Can you work these out from the model? Positions are in its coordinate system, mm. Face numbers are marked on the shaded views. A direction names the side the tool comes from. Round coordinates to 2 decimals unless told otherwise and drop trailing zeros. Loops run counter-clockwise (first coordinate to the right, second up) from the corner with the lowest first, then second, coordinate; pieces in that order, holes last. Notation, with made-up numbers: (-2, 53.25) -> (55, 53.25) arc R15 ccw to (55, 66.25) -> close; hole circle Ø2 at (-18.5, -34.5). An arc over 180 degrees is marked (long way). Answer as a JSON object with one key per item and string values.
```python
from build123d import *

# Parameters (mm, degrees)
EXTRUDE_1_DEPTH   = 10
EXTRUDE_1_2_DEPTH = 10
EXTRUDE_1_3_DEPTH = 10
SKETCH_1_3_R      = 25
SKETCH_1_3_R_2    = 7.5
SKETCH_1_3_R_3    = 5
SKETCH_1_3_R_4    = 43
SKETCH_1_3_R_5    = 6
SKETCH_1_3_R_6    = 16
EXTRUDE_2_DEPTH   = 20


with BuildPart() as part:
    # Sketch 1 → Extrude 1 (new body)
    with BuildSketch(Plane.XY):
        with BuildLine():
            ThreePointArc((105.256123955, 41.758974142), (43.471517996, 43.816308869), (-13.895789474, 20.782373178))
            ThreePointArc((-13.895789474, 20.782373178), (3.574397154, 24.743154306), (19.209372712, 16))
            ThreePointArc((19.209372712, 16), (18.448719356, 19.393999935), (20.761928319, 21.991478208))
            ThreePointArc((20.761928319, 21.991478208), (36.009186006, 26.873359096), (51.727153653, 29.915910824))
            ThreePointArc((51.727153653, 29.915910824), (57.357710528, 27.382727589), (57.596791581, 21.213203436))
            ThreePointArc((57.596791581, 21.213203436), (77.977273362, 39.487045696), (105.256123955, 41.758974142))
        make_face()
    extrude(amount=EXTRUDE_1_DEPTH)



with BuildPart() as body_2:
    # Sketch 1 → Extrude 1 2 (new body)
    with BuildSketch(Plane.XY):
        with BuildLine():
            ThreePointArc((47.755952756, -7), (51.392501916, -8.227630546), (53.540938133, -11.408163265))
            ThreePointArc((53.540938133, -11.408163265), (52, 0), (53.540938133, 11.408163265))
            ThreePointArc((53.540938133, 11.408163265), (51.392501916, 8.227630546), (47.755952756, 7))
            Line((47.755952756, 7), (28.142494559, 7))
            ThreePointArc((28.142494559, 7), (24.909599122, 7.945458765), (22.695560128, 10.483870968))
            ThreePointArc((22.695560128, 10.483870968), (24.417094455, 5.367075405), (25, 0))
            ThreePointArc((25, 0), (24.417094455, -5.367075405), (22.695560128, -10.483870968))
            ThreePointArc((22.695560128, -10.483870968), (24.909599122, -7.945458765), (28.142494559, -7))
            Line((28.142494559, -7), (47.755952756, -7))
        make_face()
    extrude(amount=EXTRUDE_1_2_DEPTH)


with BuildPart() as body_3:
    # Sketch 1 → Extrude 1 3 (new body)
    with BuildSketch(Plane.XY):
        with BuildLine():
            ThreePointArc((-54, 29), (-58.686291501, 40.313708499), (-70, 45))
            Line((-70, 45), (-70, -125))
            ThreePointArc((-70, -125), (-58.686291501, -120.313708499), (-54, -109))
            Line((-54, -109), (-54, -100.391329163))
            ThreePointArc((-54, -100.391329163), (-51.241745904, -92.047280445), (-44.053835854, -86.991089805))
            Line((-44.053835854, -86.991089805), (107.451067266, -41.15787803))
            ThreePointArc((107.451067266, -41.15787803), (81.540043629, -40.839069217), (60.517137347, -25.689145242))
            ThreePointArc((60.517137347, -25.689145242), (61.99532492, -34.793587478), (55.393464002, -41.234964608))
            Line((55.393464002, -41.234964608), (14.737358223, -53.534235903))
            ThreePointArc((14.737358223, -53.534235903), (9.423979121, -52.60916728), (7, -47.791276178))
            Line((7, -47.791276178), (7, -28.142494559))
            ThreePointArc((7, -28.142494559), (7.945458765, -24.909599122), (10.483870968, -22.695560128))
            ThreePointArc((10.483870968, -22.695560128), (0, -25), (-10.483870968, -22.695560128))
            ThreePointArc((-10.483870968, -22.695560128), (-7.945458765, -24.909599122), (-7, -28.142494559))
            Line((-7, -28.142494559), (-7, -55.656787337))
            ThreePointArc((-7, -55.656787337), (-8.182108898, -59.232808217), (-11.262641777, -61.399747063))
            Line((-11.262641777, -61.399747063), (-41.104402961, -70.427466509))
            ThreePointArc((-41.104402961, -70.427466509), (-49.960034799, -68.88568547), (-54, -60.855866967))
            Line((-54, -60.855866967), (-54, -13.5))
            ThreePointArc((-54, -13.5), (-52.242640687, -9.257359313), (-48, -7.5))
            Line((-48, -7.5), (-27.906092525, -7.5))
            ThreePointArc((-27.906092525, -7.5), (-24.718414636, -8.416820908), (-22.504913326, -10.887096774))
            ThreePointArc((-22.504913326, -10.887096774), (-25, 0), (-22.504913326, 10.887096774))
            ThreePointArc((-22.504913326, 10.887096774), (-24.718414636, 8.416820908), (-27.906092525, 7.5))
            Line((-27.906092525, 7.5), (-48, 7.5))
            ThreePointArc((-48, 7.5), (-52.242640687, 9.257359313), (-54, 13.5))
            Line((-54, 13.5), (-54, 29))
        make_face()
    extrude(amount=EXTRUDE_1_3_DEPTH)


with BuildPart() as part_1:
    add(part.part)

    add(body_2.part)  # Extrude 2 merges body 2

    add(body_3.part)  # Extrude 2 merges body 3
    # Sketch 1_3 → Extrude 2 (add)
    # profile 1 of 2: a face of its own
    with BuildSketch(Plane.XY):
        with Locations(Location((0, 0, 0), (0, 0, 154.183912666))):
            Circle(SKETCH_1_3_R)
        Circle(SKETCH_1_3_R_2, mode=Mode.SUBTRACT)
        with Locations((0, 16)):
            Circle(SKETCH_1_3_R_3, mode=Mode.SUBTRACT)
        with Locations((13.856406461, -8)):
            Circle(SKETCH_1_3_R_3, mode=Mode.SUBTRACT)
        with Locations((-13.856406461, -8)):
            Circle(SKETCH_1_3_R_3, mode=Mode.SUBTRACT)
    # profile 2 of 2: a face of its own
    with BuildSketch(Plane.XY):
        with Locations(Location((95, 0, 0), (0, 0, 164.614856568))):
            Circle(SKETCH_1_3_R_4)
        with Locations((73.786796564, 21.213203436)):
            Circle(SKETCH_1_3_R_5, mode=Mode.SUBTRACT)
        with Locations((65, 0)):
            Circle(SKETCH_1_3_R_5, mode=Mode.SUBTRACT)
        with Locations((73.786796564, -21.213203436)):
            Circle(SKETCH_1_3_R_5, mode=Mode.SUBTRACT)
        with Locations((95, -30)):
            Circle(SKETCH_1_3_R_5, mode=Mode.SUBTRACT)
        with Locations((116.213203436, -21.213203436)):
            Circle(SKETCH_1_3_R_5, mode=Mode.SUBTRACT)
        with Locations((125, 0)):
            Circle(SKETCH_1_3_R_5, mode=Mode.SUBTRACT)
        with Locations((116.213203436, 21.213203436)):
            Circle(SKETCH_1_3_R_5, mode=Mode.SUBTRACT)
        with Locations((95, 30)):
            Circle(SKETCH_1_3_R_5, mode=Mode.SUBTRACT)
        with Locations((95, 0)):
            Circle(SKETCH_1_3_R_6, mode=Mode.SUBTRACT)
    extrude(amount=EXTRUDE_2_DEPTH)


solid = part_1.part
```
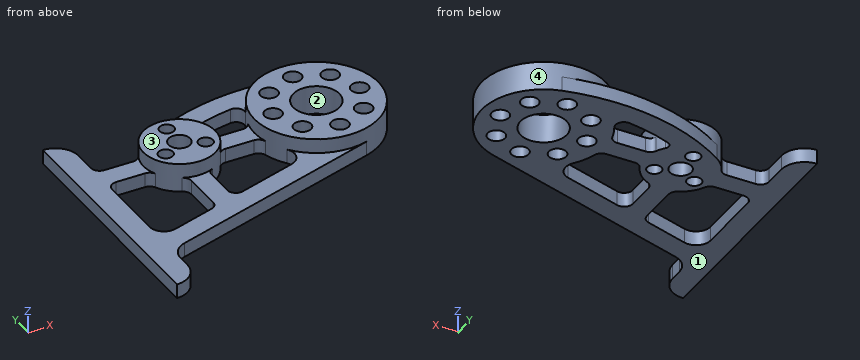
Q1. On a 3-axis mill with a long thin cutter (end or side, diameter ignored), from which of +Z, -Z, +X, -X, +Y, -Y can I reach the whole of each face in a straight line? I mean the marked faces 3 and 4. Say none if no direction works.
Determined:
{"face 3": "+Z, +X, -X, +Y, -Y", "face 4": "+Z"}
Q2. I'm going to push flat-ended pins straight in: pin 1 (11 mm diameter, centred on x = 36, z = 6.5, fed in from +Y); pin 2 (3 mm diameter, centred on x = -40.5, z = 5, fed in from +Y); pin 3 (10 mm diameter, centred on y = -13, z = 17, fed in from +X). Where does each tip first touch, or does it pass through?
Determined:
{"pin 1": "y = 43.46", "pin 2": "y = 7.5", "pin 3": "x = 137.25"}
Q3. If I drill on L1, parallel to Y at x = 95, z = 11.5; L2, parallel to Y at x = 95, z = 5; L3, parallel to Y at x = 10, z = 9.25, over which ranges is the centre line in solid material (lowest first)? Write a range as [from, to].
Determined:
{"L1": "[-43, -36], [-24, -16], [16, 24], [36, 43]", "L2": "[-44.92, -36], [-24, -16], [16, 24], [36, 43.9]", "L3": "[-70.64, -52.99], [-22.95, -11.18], [-4.82, 33.79]"}
Q4. I want a section at D-D, the plane y = -64. Write out the boundary of the cut face in (x, z), then the cut area to 3 significant figures.
Determined:
{"outline": "(-70, 0) -> (-53.49, 0) -> (-53.49, 10) -> (-70, 10) -> close; (-19.86, 0) -> (31.94, 0) -> (31.94, 10) -> (-19.86, 10) -> close", "area": "683 mm²"}
Q5. I want a section at A-A, the plane z = 15.25. Give the number of separate pieces and of enclosed holes in the cut face, then the cut area to 3 significant figures.
Determined:
{"separate pieces": "2", "enclosed holes": "13", "area": "5,650 mm²"}
Q6. I want a section at B-B, the plane y = 0. Write out the boundary of the cut face in (x, z), then the cut area to 3 significant figures.
Determined:
{"outline": "(-70, 0) -> (-7.5, 0) -> (-7.5, 20) -> (-25, 20) -> (-25, 10) -> (-70, 10) -> close; (7.5, 0) -> (59, 0) -> (59, 20) -> (52, 20) -> (52, 10) -> (25, 10) -> (25, 20) -> (7.5, 20) -> close; (71, 0) -> (79, 0) -> (79, 20) -> (71, 20) -> close; (111, 0) -> (119, 0) -> (119, 20) -> (111, 20) -> close; (131, 0) -> (138, 0) -> (138, 20) -> (131, 20) -> close", "area": "2,020 mm²"}
Q7. We'd pull the mould along Y, two halves only. Please class the marked faces 1 and 2: pulls with the +Y half, pulls with the -Y half, needs draft (parallel to the pull), parting line crosses it, or undercut.
Determined:
{"face 1": "needs draft", "face 2": "undercut"}
Q8. I want a section at C-C, the plane x = 116.5. Write out the boundary of the cut face in (y, z).
Determined:
{"outline": "(-37.24, 0) -> (-27.21, 0) -> (-27.21, 20) -> (-37.24, 20) -> close; (-15.22, 0) -> (15.22, 0) -> (15.22, 20) -> (-15.22, 20) -> close; (27.21, 0) -> (37.24, 0) -> (37.24, 20) -> (27.21, 20) -> close"}
